Design review of the part built by this model. Coordinates are the model's own, in mm. Coordinates: 2 decimals unless noted, no trailing zeros. Order: outer loops, then holes, each group sorted by start corner. A loop starts at its lowest first (then second) coordinate and runs counter-clockwise, first axis right, second up. Notation, with made-up numbers: M -12.75,59.5 L 19.25,59.5 A18 ccw 19.25,81.5 Z; hole C 67,7.25 d3. An arc over 180 degrees is marked long. Answer in a Markdown table with one row per item.
Autodesk Inventor part; units mm, degrees
ref_plane "YZ Plane" through (0, 0, 0) normal (1, 0, 0) x (0, 1, 0)
ref_plane "XZ Plane" through (0, 0, 0) normal (0, 1, 0) x (-1, 0, 0)
ref_plane "XY Plane" through (0, 0, 0) normal (0, 0, 1) x (1, 0, 0)
sketch "Sketch1" plane through (0, 0, 0) normal (0, 1, 0) x (-1, 0, 0)
  line L0 (42.2, 26.8172) -> (42.2, -26.8172)
  line L1 (0, 0) -> (0, -50) construction
  line L2 (-42.2, 26.8172) -> (-42.2, -26.8172)
  arc A0 (42.2, 26.8172) -> (-42.2, 26.8172) centre (0, 0) ccw
  arc A1 (-42.2, -26.8172) -> (42.2, -26.8172) centre (0, 0) ccw
  line L3 (39.2, 5) -> (36.7, 5)
  line L4 (36.7, 5) -> (36.7, -5)
  line L5 (36.7, -5) -> (39.2, -5)
  line L6 (39.2, -5) -> (39.2, 5)
  circle A2 centre (0, 0) radius 7.75
  line L7 (1.25, -12) -> (-1.25, -12)
  line L8 (-1.25, -12) -> (-1.25, -30)
  line L9 (-1.25, -30) -> (1.25, -30)
  line L10 (1.25, -30) -> (1.25, -12)
  line L11 (10.95, -22) -> (8.45, -22)
  line L12 (8.45, -22) -> (8.45, -34)
  line L13 (8.45, -34) -> (10.95, -34)
  line L14 (10.95, -34) -> (10.95, -22)
  line L15 (8.45, -13.6) -> (8.45, -20)
  line L16 (24.05, -20) -> (24.05, -13.6)
  line L17 (18.55, -7.2) -> (13.95, -7.2)
  line L18 (13.95, -25.2) -> (18.55, -25.2)
  line L19 (18, 37.1) -> (-4, 37.1)
  line L20 (-4, 37.1) -> (-4, 24.85)
  line L21 (-4, 24.85) -> (18, 24.85)
  line L22 (18, 24.85) -> (18, 37.1)
  line L23 (25.2374, 36.0427) -> (26.9581, 38.5001)
  line L24 (0, 0) -> (7.6405, 43.3315) construction
  line L25 (7.6405, 43.3315) -> (8.1615, 46.286)
  line L26 (0, 0) -> (42.2, 0) construction
  line L27 (25.2374, -36.0427) -> (26.9581, -38.5001)
  line L28 (7.6405, -43.3315) -> (8.1615, -46.286)
  arc A3 (7.6405, -43.3315) -> (25.2374, -36.0427) centre (0, 0) ccw
  arc A4 (25.2374, 36.0427) -> (7.6405, 43.3315) centre (0, 0) ccw
  arc A5 (8.1615, -46.286) -> (26.9581, -38.5001) centre (0, 0) ccw
  arc A6 (26.9581, 38.5001) -> (8.1615, 46.286) centre (0, 0) ccw
  line L29 (0, 0) -> (25.2374, 36.0427) construction
  line L30 (16.25, -7.2) -> (16.25, -25.2) construction
  line L31 (18.55, -25.2) -> (18.55, -20)
  line L32 (18.55, -13.6) -> (18.55, -7.2)
  line L33 (24.05, -13.6) -> (18.55, -13.6)
  line L34 (13.95, -13.6) -> (8.45, -13.6)
  line L35 (13.95, -7.2) -> (13.95, -13.6)
  line L36 (13.95, -20) -> (13.95, -25.2)
  line L37 (8.45, -20) -> (13.95, -20)
  line L38 (18.55, -20) -> (24.05, -20)
  line L39 (-39.2, 5) -> (-36.7, 5)
  line L40 (-36.7, 5) -> (-36.7, -5)
  line L41 (-36.7, -5) -> (-39.2, -5)
  line L42 (-39.2, -5) -> (-39.2, 5)
  line L43 (-8.45, 16.1) -> (-8.45, 9.2)
  line L44 (-11.55, 9.2) -> (-11.55, 16.1)
  line L45 (-10.95, -22) -> (-8.45, -22)
  line L46 (-8.45, -22) -> (-8.45, -34)
  line L47 (-8.45, -34) -> (-10.95, -34)
  line L48 (-10.95, -34) -> (-10.95, -22)
  line L49 (-8.45, -13.6) -> (-8.45, -20)
  line L50 (-24.05, -20) -> (-24.05, -13.6)
  line L51 (-18.55, -7.2) -> (-13.95, -7.2)
  line L52 (-13.95, -25.2) -> (-18.55, -25.2)
  line L53 (-25.2374, 36.0427) -> (-26.9581, 38.5001)
  line L54 (-7.6405, 43.3315) -> (-8.1615, 46.286)
  line L55 (0, 0) -> (-42.2, 0) construction
  line L56 (-25.2374, -36.0427) -> (-26.9581, -38.5001)
  line L57 (-7.6405, -43.3315) -> (-8.1615, -46.286)
  arc A7 (-25.2374, -36.0427) -> (-7.6405, -43.3315) centre (0, 0) ccw
  arc A8 (-7.6405, 43.3315) -> (-25.2374, 36.0427) centre (0, 0) ccw
  arc A9 (-26.9581, -38.5001) -> (-8.1615, -46.286) centre (0, 0) ccw
  arc A10 (-8.1615, 46.286) -> (-26.9581, 38.5001) centre (0, 0) ccw
  line L58 (-18.55, -25.2) -> (-18.55, -20)
  line L59 (-18.55, -13.6) -> (-18.55, -7.2)
  line L60 (-24.05, -13.6) -> (-18.55, -13.6)
  line L61 (-13.95, -13.6) -> (-8.45, -13.6)
  line L62 (-13.95, -7.2) -> (-13.95, -13.6)
  line L63 (-13.95, -20) -> (-13.95, -25.2)
  line L64 (-8.45, -20) -> (-13.95, -20)
  line L65 (-18.55, -20) -> (-24.05, -20)
  circle A11 centre (0, 0) radius 45.5 construction
  circle A12 centre (32.2, -32.1467) radius 1
  circle A13 centre (32.2, 11.5) radius 1
  line L66 (11.95, 11.5) -> (32.2, 11.5) construction
  circle A14 centre (32.2, -11.5) radius 1
  circle A15 centre (32.2, 32.1467) radius 1
  circle A16 centre (-32.2, -32.1467) radius 1
  circle A17 centre (-32.2, 11.5) radius 1
  circle A18 centre (-32.2, -11.5) radius 1
  circle A19 centre (-32.2, 32.1467) radius 1
  arc A20 (-8.45, 16.1) -> (-11.55, 16.1) centre (-10, 16.1) ccw
  arc A21 (-11.55, 9.2) -> (-8.45, 9.2) centre (-10, 9.2) ccw
  arc A22 (-9.8689, 7.6556) -> (-8.45, 9.2) centre (-10, 9.2) ccw
  line L67 (11.55, 9.2) -> (11.55, 16.1)
  line L68 (8.45, 16.1) -> (8.45, 9.2)
  arc A23 (11.55, 16.1) -> (8.45, 16.1) centre (10, 16.1) ccw
  arc A24 (8.45, 9.2) -> (11.55, 9.2) centre (10, 9.2) ccw
  circle A25 centre (-8.05, 20.5) radius 1.4
  circle A26 centre (8.05, 20.5) radius 1.4
  circle A27 centre (-20.65, 20.5) radius 1.4
  circle A28 centre (20.65, 20.5) radius 1.4
  line L69 (-1.55, 11.2) -> (-1.55, 18.1)
  arc A29 (1.55, 18.1) -> (-1.55, 18.1) centre (0, 18.1) ccw
  line L70 (1.55, 18.1) -> (1.55, 11.2)
  arc A30 (-1.55, 11.2) -> (1.55, 11.2) centre (0, 11.2) ccw
  circle A31 centre (0, 45.5) radius 2.5
  line L71 (0, 45.5) -> (0, 50) construction
  line L72 (0, 50) -> (0, 45.5) construction
  point P0 (-16.25, -7.2)
  point P1 (26.0977, -37.2714)
  dimension "d1" = 42.2
  dimension "d2" = 50
  dimension "d5" = 10
  dimension "d6" = 35
  dimension "d7" = 44
  dimension "d8" = 47
  dimension "d9" = 10
  dimension "d10" = 3
  dimension "d11" = 2.5
  dimension "d12" = 15.5
  dimension "d13" = 12
  dimension "d14" = 18
  dimension "d15" = 1.25
  dimension "d20" = 12
  dimension "d21" = 10
  dimension "d22" = 12.25
  dimension "d23" = 4
  dimension "d24" = 22
  dimension "d26" = 4.6
  dimension "d27" = 6.4
  dimension "d28" = 18
  dimension "d30" = 5.5
  dimension "d39" = 10
  dimension "d40" = 2
  dimension "d47" = 20.25
  dimension "d52" = 2.8
  dimension "d55" = 12.6
  dimension "d57" = 20.5
  dimension "d58" = 3.1
  dimension "d59" = 6.9
  dimension "d60" = 3.1
  dimension "d61" = 11.2
  dimension "d62" = 13.1
  dimension "d63" = 16.1
  dimension "d64" = 2
  dimension "d65" = 6.5
  dimension "d66" = 24.85
  dimension "d67" = 5.2
  dimension "d68" = 25.2
  dimension "d69" = 5
extrude "Extrusion1" add sketch "Sketch1" along normal blind 1.5 contours L0 A1 L2 A0 | L43 A21 L44 A20 | A24 L68 A23 L67 | L69 A29 L70 A30
sketch "Sketch2" plane through (0, 1.5, 0) normal (0, 1, 0) x (1, 0, 0)
  line L0 (-24.05, 13.6) -> (-24.05, 20) construction
  line L1 (24.05, 13.6) -> (24.05, 20) construction
  line L2 (24.05, 16.8) -> (49.05, 16.8) construction
  line L3 (-24.05, 16.8) -> (-24.05, -20.5) construction
  line L4 (-24.05, -20.5) -> (-49.8842, -20.5) construction
  circle A0 centre (-20.65, -20.5) radius 1.4
  line L5 (-24.05, 20) -> (-24.05, 13.6)
  line L6 (-24.05, 16.8) -> (-50.8471, 16.8) construction
  point P0 (0, 0)
properties part number "base_quick"
(1) Add section D-D, the plane z = -41. Give the boundary of the cut face in (x, y), and give its area (3 significant figures).
Return value:
| item | result |
|---|---|
| outline | M -28.62,0 L -22.98,0 L -22.98,1.5 L -28.62,1.5 Z; M -15.97,0 L 15.97,0 L 15.97,1.5 L -15.97,1.5 Z; M 22.98,0 L 28.62,0 L 28.62,1.5 L 22.98,1.5 Z |
| area | 64.8 mm2 |
(2) Add section B-B, the plane x = -20.65. Give the boundary of the cut face in (y, z).
Return value:
| item | result |
|---|---|
| outline | M 0,-45.54 L 1.5,-45.54 L 1.5,-42.22 L 0,-42.22 Z; M 0,-38.85 L 1.5,-38.85 L 1.5,-20 L 0,-20 Z; M 0,-13.6 L 1.5,-13.6 L 1.5,19.1 L 0,19.1 Z; M 0,21.9 L 1.5,21.9 L 1.5,38.85 L 0,38.85 Z; M 0,42.22 L 1.5,42.22 L 1.5,45.54 L 0,45.54 Z |
(3) Add section C-C, the plane z = 0. Give the boundary of the cut face in (x, y), and give its area (4 significant figures).
Return value:
| item | result |
|---|---|
| outline | M -42.2,0 L -39.2,0 L -39.2,1.5 L -42.2,1.5 Z; M -36.7,0 L -7.75,0 L -7.75,1.5 L -36.7,1.5 Z; M 7.75,0 L 36.7,0 L 36.7,1.5 L 7.75,1.5 Z; M 39.2,0 L 42.2,0 L 42.2,1.5 L 39.2,1.5 Z |
| area | 95.85 mm2 |
(4) Add section A-A, the plane z = 20.5. Give the boundary of the cut face in (x, y), and give its area (3 significant figures).
Return value:
| item | result |
|---|---|
| outline | M -42.2,0 L -22.05,0 L -22.05,1.5 L -42.2,1.5 Z; M -19.25,0 L -9.45,0 L -9.45,1.5 L -19.25,1.5 Z; M -6.65,0 L 6.65,0 L 6.65,1.5 L -6.65,1.5 Z; M 9.45,0 L 19.25,0 L 19.25,1.5 L 9.45,1.5 Z; M 22.05,0 L 42.2,0 L 42.2,1.5 L 22.05,1.5 Z |
| area | 110 mm2 |
(5) For line 1 along X through (y, z) = (0.15, -21); line 2 along X through (y, z) = (0.4, -24); line 3 along X through (y, z) = (0.8, 0.5), list the stretches that pass through material, from the lowest coordinate up. Write a range as from..to.
Return value:
| item | result |
|---|---|
| line 1 | x = -42.2..-18.55, -13.95..-1.25, 1.25..13.95, 18.55..42.2 |
| line 2 | x = -42.2..-18.55, -13.95..-10.95, -8.45..-1.25, 1.25..8.45, 10.95..13.95, 18.55..42.2 |
| line 3 | x = -42.2..-39.2, -36.7..-7.73, 7.73..36.7, 39.2..42.2 |
(6) Insertion check: pin 1 Ø0.8 at (x, y) = (22.5, 1) entering from +Z; pin 2 Ø0.8 at (x, y) = (0, 1) entering from +Z. Each pin has a flat end and moves straight along its axis. Give the tip position at first contact, or say it passes through.
Return value:
| item | result |
|---|---|
| pin 1 | stops at z = 44.85 |
| pin 2 | stops at z = 50 |
(7) Draft analysis for pull direction Z (two halves, no side actions). For faces 1 (the flat face through (10, 0, 1)), 2 (the cylindrical face through (-0.703, 0.74, -49.995)), 3 (the cylindrical face through (-17.85, 0.74, 43.48)), state which applies: pulls with the +Z half, pulls with the -Z half, needs draft (parallel to the pull), parting line crosses it, or undercut.
Return value:
| item | result |
|---|---|
| face 1 | needs draft |
| face 2 | pulls with the -Z half |
| face 3 | undercut |
